Source: CAD feature listing. Evaluate the final solid. Frame: model axes, mm. A direction names the side the tool comes from. Coordinates: 2 decimals unless noted, no trailing zeros. Write each loop counter-clockwise with the first axis right and the second up, starting at its lowest first coordinate (ties: lowest second). Pieces come first, ordered by that corner, then holes. Notation, with made-up numbers: (75, 70) -> (116, 70) arc R13 ccw to (116, 76) -> close; hole circle Ø11 at (-32, 66.5). An arc over 180 degrees is marked (long way). One line per item, written item: value. Start each with the question number.
1. Mould query, pull axis X, two halves, no side actions, for faces 4 (the flat face through (22, 16, 25.4)), 5 (the flat face through (66.13, 12.61, 17.71)), 6 (the flat face through (38, 26, 12.7)), 7 (the flat face through (46.99, 25, 18)). Classes: released by +X, released by -X, zero draft, split by the parting line, or undercut.
2. Access query for faces 1 (the flat face through (34, 6.35, 18)), 2 (the flat face through (53.25, 12.79, 17.71)), 3 (the flat face through (41.8, 33.04, 24.15)). Directions: +Z, -Z, +X, -X, +Y, -Y. A direction counts if a zero-diameter tool reaches every point of the face in a straight line with its end or side. Return the directions, or none.
3. Section query C-C, the plane y = 43.5. Output: boundary loops of the cut face in (x, z).
4. Section query A-A, the plane z = 13.75. Output: boundary loops of the cut face in (x, y).
5. First-contact query: P1, Ø12, axis at x = 24.5, z = 20, coming from the +Y side; P2, Ø8, axis at x = 33.5, z = 17.5, coming from the -Y side; P3, Ø3, axis at y = 24, z = 15.5, coming from the +X side. Flat tips, straight axial feed; report the tip coordinate or a pass-through.
6. Line query: line 1 (X direction, y = 22, z = 19); line 2 (Z direction, x = 45, y = 31); line 3 (X direction, y = 38.5, z = 22.25). Output: solid intervals per line, ascending.
7. Section query B-B, the plane x = 38.5. Output: boundary loops of the cut face in (y, z).
8. Section query D-D, the plane y = 14. Output: boundary loops of the cut face in (x, z).
from build123d import *

# Parameters (mm, degrees)
F0_W     = 76.2
F0_H     = 50.8
F1_DEPTH = 25.4
F2_W     = 76.2
F2_H     = 50.8
F3_DEPTH = 12.7
F5_DEPTH = 12.7
F6_SIZE  = 2.54


with BuildPart() as f1:
    # F0 (on Top) → F1 (new body)
    with BuildSketch(Plane.XY):
        with Locations((38.1, 25.4)):
            Rectangle(F0_W, F0_H)
    extrude(amount=F1_DEPTH)

    # F2 (on face) → F3 (cut)
    with BuildSketch(Plane.XY.offset(25.4)):
        with Locations((38.1, 25.4)):
            Rectangle(F2_W, F2_H)
    extrude(amount=-F3_DEPTH, mode=Mode.SUBTRACT)

    # F4 (on face) → F5 (join)
    with BuildSketch(Plane.XY.offset(12.7)):
        Polygon((21.59, 31.75), (8.89, 44.45), (8.89, 31.75), (8.89, 19.05), (21.59, 6.35), (34.29, 6.35), (46.99, 6.35), (34.29, 19.05), (21.59, 19.05), align=None)
        Polygon((46.99, 19.05), (59.69, 6.35), (72.39, 6.35), (59.69, 19.05), (59.69, 31.75), (46.99, 44.45), (34.29, 44.45), (21.59, 44.45), (34.29, 31.75), (46.99, 31.75), align=None)
    extrude(amount=F5_DEPTH)

    # F6
    f6_edges = [f1.edges().sort_by_distance(p)[0] for p in [
        (15.24, 12.7, 25.4),
        (8.89, 31.75, 25.4),
        (15.24, 38.1, 25.4),
        (21.59, 25.4, 25.4),
        (27.94, 19.05, 25.4),
        (40.64, 12.7, 25.4),
        (34.29, 6.35, 25.4),
        (53.34, 12.7, 25.4),
        (66.04, 12.7, 25.4),
        (66.04, 6.35, 25.4),
        (46.99, 25.4, 25.4),
        (53.34, 38.1, 25.4),
        (27.94, 38.1, 25.4),
        (34.29, 44.45, 25.4),
        (40.64, 31.75, 25.4),
        (59.69, 25.4, 25.4),
    ]]
    chamfer(f6_edges, length=F6_SIZE)


solid = f1.part
Computed values:
1. face 4: zero draft
1. face 5: released by +X
1. face 6: undercut
1. face 7: undercut
2. face 1: +Z, +X, -X, -Y
2. face 2: +Z, -Y
2. face 3: +Z
3. outline: (0, 0) -> (76.2, 0) -> (76.2, 12.7) -> (47.94, 12.7) -> (47.94, 22.86) -> (46.6, 23.81) -> (23.88, 23.81) -> (22.54, 22.86) -> (22.54, 12.7) -> (9.84, 12.7) -> (9.84, 22.86) -> (9.28, 23.25) -> (8.89, 22.86) -> (8.89, 12.7) -> (0, 12.7) -> close
4. outline: (8.89, 19.05) -> (21.59, 6.35) -> (46.99, 6.35) -> (34.29, 19.05) -> (21.59, 19.05) -> (21.59, 31.75) -> (8.89, 44.45) -> close; (21.59, 44.45) -> (34.29, 31.75) -> (46.99, 31.75) -> (46.99, 19.05) -> (59.69, 6.35) -> (72.39, 6.35) -> (59.69, 19.05) -> (59.69, 31.75) -> (46.99, 44.45) -> close
5. P1: stops at y = 44.45
5. P2: stops at y = 6.35
5. P3: stops at x = 59.69
6. line 1: x = 8.89 to 21.59, 46.99 to 59.69
6. line 2: z = 0 to 12.7
6. line 3: x = 8.89 to 14.84, 27.54 to 52.94
7. outline: (0, 0) -> (50.8, 0) -> (50.8, 12.7) -> (44.45, 12.7) -> (44.45, 22.86) -> (41.91, 25.4) -> (34.29, 25.4) -> (31.75, 22.86) -> (31.75, 12.7) -> (14.84, 12.7) -> (14.84, 22.86) -> (11.25, 25.4) -> (8.89, 25.4) -> (6.35, 22.86) -> (6.35, 12.7) -> (0, 12.7) -> close
8. outline: (0, 0) -> (76.2, 0) -> (76.2, 12.7) -> (64.74, 12.7) -> (64.74, 22.86) -> (61.15, 25.4) -> (55.63, 25.4) -> (52.04, 22.86) -> (52.04, 12.7) -> (39.34, 12.7) -> (39.34, 22.86) -> (35.75, 25.4) -> (17.53, 25.4) -> (13.94, 22.86) -> (13.94, 12.7) -> (0, 12.7) -> close
